Read the model definition and answer for the solid it produces. Units are mm, in the model's axes. A direction names the side the tool comes from. Round coordinates to 2 decimals unless told otherwise and drop trailing zeros. Write each loop counter-clockwise with the first axis right and the second up, starting at its lowest first coordinate (ties: lowest second). Pieces come first, ordered by that corner, then holes. Notation, with made-up numbers: (5.5, 42.5) - (13.5, 42.5) arc R28 ccw to (13.5, 60.5) - close; hole circle Ø8 at (16, 5). An arc over 180 degrees is marked (long way). One line per item, written item: value. Start each with the question number.
(1) For faces 1 (the face through (-4.246, -9.619, 16.48)), 2 (the face through (4.246, -33.146, 9.455)), 3 (the face through (-13.64, -25.113, 24.461)), 4 (the face through (-13.925, -14, 14)), 5 (the face through (0.093, -25.117, 12.418)), determine the directions among +Z, -Z, +X, -X, +Y, -Y from which every point of the face is accessible in a straight line to the end or side of a thin tool.
(2) Find the intervals of material crossed by L1, parallel to Y at x = 0, z = 2.55; L2, parallel to Y at x = 2, z = 5.5; L3, parallel to X at y = -33, z = 6.5 (3 decimals), in increasing order.
(3) Flat-ended cylindrical pins translate along their axes: pin 1 Ø13.5 at (x, y) = (0, -33.33) entering from +Z; pin 2 Ø1.5 at (x, z) = (4.5, 20.5) entering from -Y; pin 3 Ø2.5 at (x, y) = (2, -16) entering from +Z. Find the tip coordinate at first contact, or state that the pin passes through.
(4) A cutting plane is placed at A-A, the plane x = 0. State how many separate pieces and enclosed holes the cut face has, plus the area to 3 significant figures.
(5) A cutting plane is placed at B-B, the plane x = -3.5. Determine the outline of the cut face in (y, z), plus the area to 3 significant figures.
(6) The mould has two halves that part along Y. Classify faces 6 (the face through (-13.64, -1.227, 1.199)), 7 (the face through (-4.25, -23, 23)), 8 (the face through (4.246, -16.48, 9.455)), 9 (the face through (0.181, -0.602, 48.503)): +Y half, -Y half, draft (parallel to the pull), parting line (faces both ways), or undercut.
(7) A cutting plane is placed at C-C, the plane x = 5. Determine the outline of the cut face in (y, z), plus the area to 3 significant figures.
from build123d import *

# Parameters (mm, degrees)
BOSS_EXTRUDE1_DEPTH  = 13.925
M4_CLEARANCE_HOLE1_D = 4.5
CUT_EXTRUDE1_START   = -5
SKETCH7_R            = 4.25
CUT_EXTRUDE1_DEPTH   = 62
CHAMFER1_SIZE        = 2
MIRROR1_START        = -33.333333
MIRROR1_OUTLINE_R    = 4.25
MIRROR1_DEPTH        = 28.333333
MIRROR1_START_2      = -5
MIRROR1_2_OUTLINE_R  = 2.25
MIRROR1_2_DEPTH      = 5
CUT_EXTRUDE4_START   = -18.175
CUT_EXTRUDE4_DEPTH   = 8.5
FILLET1_R            = 1


# Read off the part's stored shape, not the designer's step: Mirror1
with BuildPart() as part:
    # Sketch1 → Boss-Extrude1 (new, symmetric)
    with BuildSketch(Plane(origin=(0, 0, 0), x_dir=(0, 0, -1), z_dir=(1, 0, 0))):
        Polygon((0, 0), (-50, 0), (0, -50), align=None)
    extrude(amount=BOSS_EXTRUDE1_DEPTH, both=True)

    # M4 Clearance Hole1 (through all)
    with Locations(Plane(origin=(0, 0, 0), x_dir=(-1, 0, 0), z_dir=(0, 0, -1))):
        with Locations((0, -16.666667), (0, -33.333333)):
            Hole(M4_CLEARANCE_HOLE1_D / 2)

    # Sketch7 → Cut-Extrude1 (cut)
    with BuildSketch(Plane(origin=(0, 0, 0), x_dir=(-1, 0, 0), z_dir=(0, 0, -1)).offset(CUT_EXTRUDE1_START)):
        with Locations((0, -16.666667)):
            Circle(SKETCH7_R)
        with Locations((0, -33.333333)):
            Circle(SKETCH7_R)
    extrude(amount=-CUT_EXTRUDE1_DEPTH, mode=Mode.SUBTRACT)

    # Chamfer1
    chamfer1_edges = [part.edges().sort_by_distance(p)[0] for p in [
        (0, 0, 0),
    ]]
    chamfer(chamfer1_edges, length=CHAMFER1_SIZE)

    # Mirror1 outline → Mirror1 (cut)
    with BuildSketch(Plane(origin=(0, 0, 0), x_dir=(1, 0, 0), z_dir=(0, 1, 0)).offset(MIRROR1_START)):
        with Locations((0, -33.333333)):
            Circle(MIRROR1_OUTLINE_R)
        with Locations((0, -16.666667)):
            Circle(MIRROR1_OUTLINE_R)
    extrude(amount=MIRROR1_DEPTH, mode=Mode.SUBTRACT)

    # Mirror1 2 outline → Mirror1 2 (cut)
    with BuildSketch(Plane(origin=(0, 0, 0), x_dir=(1, 0, 0), z_dir=(0, 1, 0)).offset(MIRROR1_START_2)):
        with Locations((0, -33.333333)):
            Circle(MIRROR1_2_OUTLINE_R)
        with Locations((0, -16.666667)):
            Circle(MIRROR1_2_OUTLINE_R)
    extrude(amount=MIRROR1_2_DEPTH, mode=Mode.SUBTRACT)

    # Sketch8 → Cut-Extrude4 (cut)
    with BuildSketch(Plane(origin=(13.925, 0, 0), x_dir=(0, 0, -1), z_dir=(1, 0, 0)).offset(CUT_EXTRUDE4_START)):
        Polygon((-33.333333, -16.666667), (-16.666667, -16.666667), (-16.666667, -33.333333), align=None)
    extrude(amount=CUT_EXTRUDE4_DEPTH, mode=Mode.SUBTRACT)

    # Fillet1
    fillet1_edges = [part.edges().sort_by_distance(p)[0] for p in [
        (13.925, -25, 25),
        (-13.925, 0, 26),
        (13.925, 0, 26),
        (-13.925, -1, 1),
        (-13.925, -25, 25),
        (13.925, -1, 1),
        (-13.925, -26, 0),
        (13.925, -26, 0),
        (0, -50, 0),
        (0, 0, 50),
    ]]
    fillet(fillet1_edges, radius=FILLET1_R)


solid = part.part
Here are the results:
1. face 1: -Y
1. face 2: +Z
1. face 3: +Z, -X, -Y
1. face 4: +Z, -Z, -X, +Y, -Y
1. face 5: +Z, -Y
2. L1: -47.45 to -35.58, -31.08 to -18.92, -14.42 to 0
2. L2: -44.5 to -37.08, -29.58 to -20.42, -12.92 to 0
2. L3: -13.925 to -4.237, 4.237 to 13.925
3. pin 1: z = 21.91
3. pin 2: y = -30.25
3. pin 3: z = 5
4. separate pieces: 5
4. enclosed holes: 0
4. area: 587 mm²
5. outline: (-48.29, 1.71) arc R1 ccw to (-47.59, 0) - (-2, 0) - (0, 2) - (0, 47.59) arc R1 ccw to (-1.71, 48.29) - (-14.26, 35.74) - (-5, 35.74) - (-5, 30.92) - (-14.26, 30.92) - (-14.26, 19.08) - (-5, 19.08) - (-5, 14.26) - (-14.26, 14.26) - (-14.26, 5) - (-19.08, 5) - (-19.08, 14.26) - (-30.92, 14.26) - (-30.92, 5) - (-35.74, 5) - (-35.74, 14.26) - close
5. area: 836 mm²
6. face 6: +Y half
6. face 7: draft
6. face 8: undercut
6. face 9: parting line
7. outline: (-48.29, 1.71) arc R1 ccw to (-47.59, 0) - (-2, 0) - (0, 2) - (0, 47.59) arc R1 ccw to (-1.71, 48.29) - close
7. area: 1,250 mm²
